Here's how the part is built. I have some questions about the finished solid (model axes, mm). A direction names the side the tool comes from. Coordinates: 2 decimals unless noted, no trailing zeros. Write each loop counter-clockwise with the first axis right and the second up, starting at its lowest first coordinate (ties: lowest second). Pieces come first, ordered by that corner, then holes. Notation, with made-up numbers: M 33,13.5 L 39,13.5 A16 ccw 39,42.5 Z; hole C 41.25,-26.75 d1. An arc over 180 degrees is marked long. Use a Markdown table: item, result.
```python
from build123d import *

# Parameters (mm, degrees)
SKETCH_1_R      = 35
EXTRUDE_1_DEPTH = 42
SKETCH_2_R      = 3
EXTRUDE_2_DEPTH = 8


with BuildPart() as part:
    # Эскиз1 → Бобышка-Вытянуть1 (new body)
    with BuildSketch(Plane(origin=(0, 0, 0), x_dir=(1, 0, 0), z_dir=(0, 1, 0))):
        Circle(SKETCH_1_R)
    extrude(amount=EXTRUDE_1_DEPTH)

    # Эскиз2 → Бобышка-Вытянуть2 (add)
    with BuildSketch(Plane(origin=(0, 42, 0), x_dir=(1, 0, 0), z_dir=(0, 1, 0))):
        with BuildLine():
            ThreePointArc((-47, -34.641016151), (0, -47.234628196), (47, -34.641016151))
            ThreePointArc((47, -34.641016151), (51.758330249, -29.882685902), (53.5, -23.382685902))
            ThreePointArc((53.5, -23.382685902), (40.906387956, 23.617314098), (6.5, 58.023702054))
            ThreePointArc((6.5, 58.023702054), (0, 59.765371804), (-6.5, 58.023702054))
            ThreePointArc((-6.5, 58.023702054), (-40.906387956, 23.617314098), (-53.5, -23.382685902))
            ThreePointArc((-53.5, -23.382685902), (-51.758330249, -29.882685902), (-47, -34.641016151))
        make_face()
        with Locations((0, 46.765371804)):
            Circle(SKETCH_2_R, mode=Mode.SUBTRACT)
        with Locations((-40.5, -23.382685902)):
            Circle(SKETCH_2_R, mode=Mode.SUBTRACT)
        with Locations((40.5, -23.382685902)):
            Circle(SKETCH_2_R, mode=Mode.SUBTRACT)
    extrude(amount=-EXTRUDE_2_DEPTH)

    # Эскиз3 → Повернуть1 (revolve)
    with BuildSketch(Plane(origin=(0, 0, 0), x_dir=(0, 0, -1), z_dir=(1, 0, 0))):
        with BuildLine():
            Line((11, 81), (26.5, 42))
            Line((26.5, 42), (0, 42))
            Line((0, 42), (0, 128))
            ThreePointArc((0, 128), (12.02081528, 123.02081528), (17, 111))
            ThreePointArc((17, 111), (15.485292704, 95.702941459), (11, 81))
        make_face()
    revolve(axis=Axis((0, 128, 0), (0, -1, 0)))


solid = part.part
```
1. I need wall thicknesses on probe 1 along Y at (x, z) = (46.5, 25); probe 2 along Z at (x, y) = (0, 36); probe 3 along Z at (x, y) = (40.5, 37.25). Which ranges of each line are inside material? Lowest first, please.
Answers follow:
| item | result |
|---|---|
| probe 1 | y = 34 to 42 |
| probe 2 | z = -59.77 to -49.77, -43.77 to 47.23 |
| probe 3 | z = -24.31 to 20.38, 26.38 to 38.06 |
2. Will these pins go through, and if not, where does the flat tip stop? pin 1 Ø8 at (x, y) = (23, 94) entering from -Z; pin 2 Ø10 at (x, z) = (32, -38) entering from +Y; pin 3 Ø1.5 at (y, z) = (43, 6.5) entering from +X; pin 4 Ø1.5 at (x, y) = (-8.5, 98) entering from -Z.
Answers follow:
| item | result |
|---|---|
| pin 1 | passes through |
| pin 2 | stops at y = 42 |
| pin 3 | stops at x = 25.64 |
| pin 4 | stops at z = -13.92 |
3. Suppose I cut it at A-A on x = 40.5. Write out the boundary of the cut face in (y, z), and give its area (3 significant figures).
Answers follow:
| item | result |
|---|---|
| outline | M 34,-24.31 L 42,-24.31 L 42,20.38 L 34,20.38 Z; M 34,26.38 L 42,26.38 L 42,38.06 L 34,38.06 Z |
| area | 451 mm2 |
4. Suppose I cut it at B-B on z = -33. Write out the boundary of the cut face in (x, y).
Answers follow:
| item | result |
|---|---|
| outline | M -34.71,34 L -11.66,34 L -11.66,0 L 11.66,0 L 11.66,34 L 34.71,34 L 34.71,42 L -34.71,42 Z |
5. Which directions (+Z, -Z, +X, -X, +Y, -Y) give clear straight access to the entire face, cutting with the end or side of a thin tool? Please do faces 1 (the face through (35, 34, 5)), 2 (the face through (-0.689, 38.056, 47.232)), 3 (the face through (23, 42, 17)), 4 (the face through (-10.4, 65.6, 13.6)), 5 (the face through (0, 0, 0)).
Answers follow:
| item | result |
|---|---|
| face 1 | -Y |
| face 2 | +Z, +Y, -Y |
| face 3 | +Y |
| face 4 | none |
| face 5 | +Z, -Z, +X, -X, -Y |
6. Suppose I cut it at D-D on z = 39.5. Write out the boundary of the cut face in (x, y), and give its area (3 significant figures).
Answers follow:
| item | result |
|---|---|
| outline | M -37.34,34 L 37.34,34 L 37.34,42 L -37.34,42 Z |
| area | 597 mm2 |
7. We'd pull the mould along X, two halves only. Please class faces 6 (the face through (37.5, 38.1, 23.3)), 7 (the face through (51.71, 38.056, 29.965)), 8 (the face through (0.095, 38.056, -59.765)): +X half, -X half, draft (parallel to the pull), parting line (faces both ways), or undercut.
Answers follow:
| item | result |
|---|---|
| face 6 | undercut |
| face 7 | +X half |
| face 8 | parting line |
8. Suppose I cut it at C-C on y = 22.5. Write out the boundary of the cut face in (x, z), and give its area (3 significant figures).
Answers follow:
| item | result |
|---|---|
| outline | C 0,0 d70 |
| area | 3,850 mm2 |
